Here's the drawing with two shaded views (mm, measured from the low corner). I have some questions. Coordinates: 2 decimals unless noted, no trailing zeros. Write each loop counter-clockwise with the first axis right and the second up, starting at its lowest first coordinate (ties: lowest second). Pieces come first, ordered by that corner, then holes. Notation, with made-up numbers: (78, 68.25) -> (102, 68.25) arc R24 ccw to (102, 98.25) -> close; hole circle Ø7 at (-35, 50). An arc over 180 degrees is marked (long way). Put each result on its own line as item: value. Start each with the question number.
Item 1: I need wall thicknesses on line 1 (X direction, y = 7.25, z = 105); line 2 (Z direction, x = 15, y = 7.75); line 3 (X direction, y = 13.5, z = 111). Which ranges of each line are inside material? Lowest first, please. Write a range as [from, to].
Item 2: I want a section at B-B, the plane y = 18. List the corners of the cut face in (x, z) for me, then the cut area to 3 significant figures.
Item 3: I want a section at C-C, the plane x = 26. List the corners of the cut face in (y, z) for me, then the cut area to 3 significant figures.
Item 4: If we mould it in two halves opening along Z, with no side actions, what happens to the marked faces 1, 2, 3 and 4? For each: released by +Z, released by -Z, zero draft, split by the parting line, or undercut.
Item 5: I want a section at A-A, the plane x = 139. List the corners of the cut face in (y, z) for me, then the cut area to 3 significant figures.
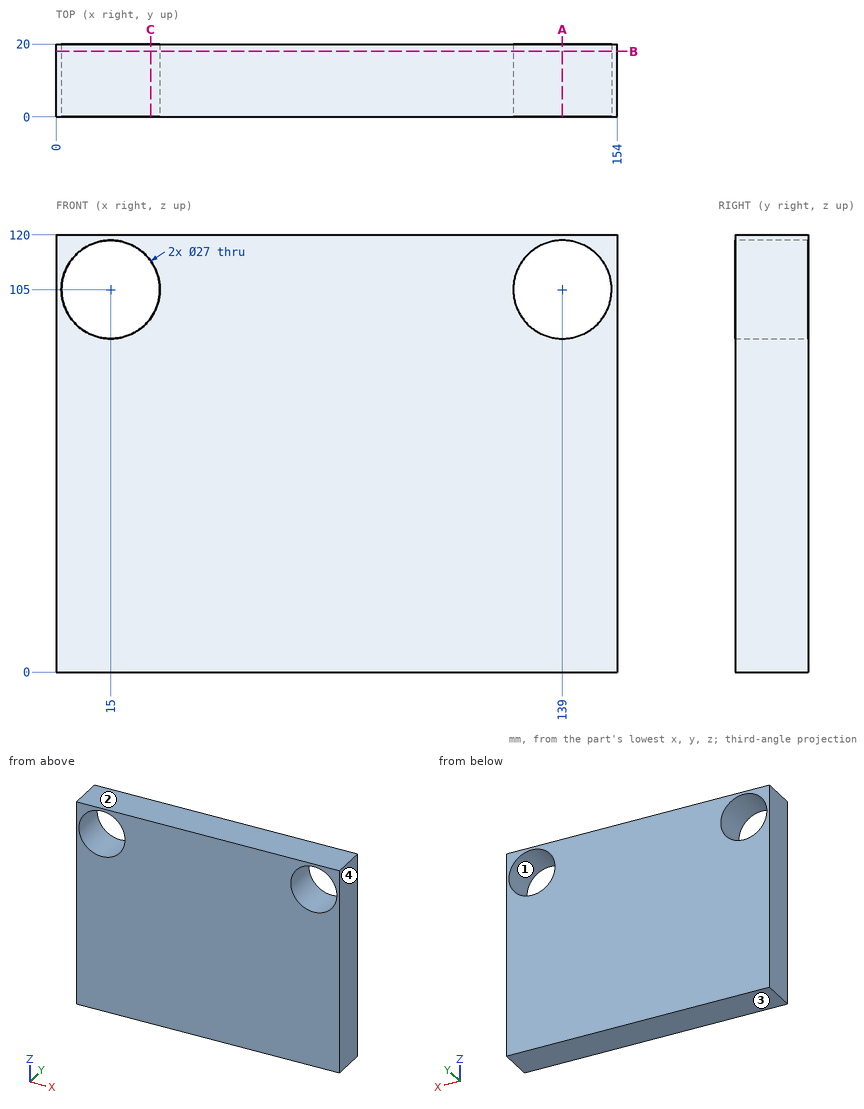
Calculated:
1. line 1: x = [0, 1.5], [28.5, 125.5], [152.5, 154]
1. line 2: z = [0, 91.5], [118.5, 120]
1. line 3: x = [0, 2.91], [27.09, 126.91], [151.09, 154]
2. outline: (0, 0) -> (154, 0) -> (154, 120) -> (0, 120) -> close; hole circle Ø27 at (15, 105); hole circle Ø27 at (139, 105)
2. area: 17,300 mm2
3. outline: (0, 0) -> (20, 0) -> (20, 97.17) -> (0, 97.17) -> close; (0, 112.83) -> (20, 112.83) -> (20, 120) -> (0, 120) -> close
3. area: 2,090 mm2
4. face 1: undercut
4. face 2: released by +Z
4. face 3: released by -Z
4. face 4: zero draft
5. outline: (0, 0) -> (20, 0) -> (20, 91.5) -> (0, 91.5) -> close; (0, 118.5) -> (20, 118.5) -> (20, 120) -> (0, 120) -> close
5. area: 1,860 mm2
